Source: CAD feature listing. Evaluate the final solid. Frame: model axes, mm. A direction names the side the tool comes from. Round coordinates to 2 decimals unless told otherwise and drop trailing zeros. Order: outer loops, then holes, each group sorted by start corner. A loop starts at its lowest first (then second) coordinate and runs counter-clockwise, first axis right, second up. Notation, with made-up numbers: (30.25, 56) - (34.25, 56) arc R20 cw to (34.25, 60) - close; hole circle Ø10 at (75.5, 85.25). An arc over 180 degrees is marked (long way). Put each result on its own line as item: value. Start each with the question number.
1) Section A-A on z = 1.5. Output: boundary loops of the cut face in (x, y).
2) Access query for faces 4 (the face through (10, 25, 1)), 5 (the face through (119, 15, 5)), 6 (the face through (51, 41, 3)). Directions: +Z, -Z, +X, -X, +Y, -Y. A direction counts if a zero-diameter tool reaches every point of the face in a straight line with its end or side. Return the directions, or none.
3) Line query: probe 1 along Y at (x, z) = (174, 8.65); probe 2 along Y at (x, z) = (50, 7.75); probe 3 along X at (y, z) = (41, 4.75). Output: solid intervals per line, ascending. Write a range as [from, to].
4) Section C-C on x = 120. Output: boundary loops of the cut face in (y, z), then the cut area to 3 significant figures.
5) Section B-B on y = 26.5. Output: boundary loops of the cut face in (x, z).
6) Mould query, pull axis X, two halves, no side actions, for faces 1 (the face through (60, 41, 5)), 2 (the face through (50, 11, 1)), 3 (the face through (116, 20.5, 2)). Classes: +X half, -X half, draft (parallel to the pull), parting line (faces both ways), or undercut.
7) Section D-D on y = 42.5. Output: boundary loops of the cut face in (x, z).
8) Contact query for flat-ended pins moving along their axis: P1, Ø1.5, axis at x = 8, y = 41.5, coming from the +Z side; P2, Ø2.5, axis at x = 109, z = 2, coming from the +Y side; P3, Ø0.9, axis at x = 140, z = 1, coming from the -Y side; P4, Ø9.5, axis at x = 10, y = 9, coming from the +Z side. Output: stop coordinate, or through.
```python
from build123d import *

# Parameters (mm, degrees)
BOSS_EXTRUDE1_DEPTH = 10
SKETCH2_R           = 3
CUT_EXTRUDE1_DEPTH  = 7
SKETCH4_W           = 40
SKETCH4_H           = 40
CUT_EXTRUDE3_DEPTH  = 3
SKETCH5_R           = 1
SKETCH5_R_2         = 4
CUT_EXTRUDE4_DEPTH  = 11
SKETCH6_W           = 3
SKETCH6_H           = 3
CUT_EXTRUDE5_DEPTH  = 130
FILLET1_R           = 2
SKETCH7_R           = 1.2
CUT_EXTRUDE6_DEPTH  = 36


with BuildPart() as part:
    # Sketch1 → Boss-Extrude1 (new body)
    with BuildSketch(Plane.XY):
        Polygon((0, 0), (60, 0), (60, 15), (180, 15), (180, 35), (60, 35), (60, 50), (0, 50), align=None)
    extrude(amount=BOSS_EXTRUDE1_DEPTH)

    # Sketch2 → Cut-Extrude1 (cut)
    with BuildSketch(Plane.XY.offset(10)):
        with Locations((10, 9)):
            Circle(SKETCH2_R)
        with Locations((50, 9)):
            Circle(SKETCH2_R)
        with Locations((50, 41)):
            Circle(SKETCH2_R)
        with Locations((10, 41)):
            Circle(SKETCH2_R)
    extrude(amount=-CUT_EXTRUDE1_DEPTH, mode=Mode.SUBTRACT)

    # Sketch4 → Cut-Extrude3 (cut)
    with BuildSketch(Plane(origin=(0, 0, 0), x_dir=(-1, 0, 0), z_dir=(0, 0, -1))):
        with Locations((-30, 25)):
            Rectangle(SKETCH4_W, SKETCH4_H)
    extrude(amount=-CUT_EXTRUDE3_DEPTH, mode=Mode.SUBTRACT)

    # Sketch5 → Cut-Extrude4 (cut, through all)
    with BuildSketch(Plane(origin=(0, 0, 0), x_dir=(-1, 0, 0), z_dir=(0, 0, -1))):
        with Locations((-174, 31)):
            Circle(SKETCH5_R)
        with Locations((-174, 19)):
            Circle(SKETCH5_R)
        with Locations((-120, 25)):
            Circle(SKETCH5_R_2)
    extrude(amount=-CUT_EXTRUDE4_DEPTH, mode=Mode.SUBTRACT)

    # Sketch6 → Cut-Extrude5 (cut)
    with BuildSketch(Plane(origin=(180, 0, 0), x_dir=(0, 0, -1), z_dir=(1, 0, 0))):
        with Locations((-1.5, 31)):
            Rectangle(SKETCH6_W, SKETCH6_H)
        with Locations((-1.5, 19)):
            Rectangle(SKETCH6_W, SKETCH6_H)
    extrude(amount=-CUT_EXTRUDE5_DEPTH, mode=Mode.SUBTRACT)

    # Fillet1
    fillet1_edges = [part.edges().sort_by_distance(p)[0] for p in [
        (0, 50, 5),
        (60, 50, 5),
        (60, 0, 5),
        (0, 0, 5),
    ]]
    fillet(fillet1_edges, radius=FILLET1_R)

    # Sketch7 → Cut-Extrude6 (cut, through all)
    with BuildSketch(Plane(origin=(0, 35, 0), x_dir=(1, 0, 0), z_dir=(0, 1, 0))):
        with Locations((174, -6)):
            Circle(SKETCH7_R)
    extrude(amount=-CUT_EXTRUDE6_DEPTH, mode=Mode.SUBTRACT)


solid = part.part
```
Answer sheet:
1. outline: (0, 2) arc R2 ccw to (2, 0) - (58, 0) arc R2 ccw to (60, 2) - (60, 15) - (180, 15) - (180, 17.5) - (50, 17.5) - (50, 5) - (10, 5) - (10, 45) - (50, 45) - (50, 32.5) - (180, 32.5) - (180, 35) - (60, 35) - (60, 48) arc R2 ccw to (58, 50) - (2, 50) arc R2 ccw to (0, 48) - close; (50, 20.5) - (180, 20.5) - (180, 29.5) - (50, 29.5) - close; hole circle Ø8 at (120, 25)
2. face 4: -Z
2. face 5: +Z, -Z, +X, -Y
2. face 6: +Z
3. probe 1: [15, 18], [20, 30], [32, 35]
3. probe 2: [0, 6], [12, 38], [44, 50]
3. probe 3: [0, 7], [13, 47], [53, 60]
4. outline: (15, 0) - (17.5, 0) - (17.5, 3) - (20.5, 3) - (20.5, 0) - (21, 0) - (21, 10) - (15, 10) - close; (29, 0) - (29.5, 0) - (29.5, 3) - (32.5, 3) - (32.5, 0) - (35, 0) - (35, 10) - (29, 10) - close
4. area: 102 mm^2
5. outline: (0, 0) - (10, 0) - (10, 3) - (50, 3) - (50, 0) - (116.29, 0) - (116.29, 10) - (0, 10) - close; (123.71, 0) - (180, 0) - (180, 10) - (123.71, 10) - close; hole circle Ø2.4 at (174, 6)
6. face 1: +X half
6. face 2: undercut
6. face 3: draft
7. outline: (0, 0) - (10, 0) - (10, 3) - (7.4, 3) - (7.4, 10) - (0, 10) - close; (12.6, 3) - (47.4, 3) - (47.4, 10) - (12.6, 10) - close; (50, 0) - (60, 0) - (60, 10) - (52.6, 10) - (52.6, 3) - (50, 3) - close
8. P1: z = 3
8. P2: y = 35
8. P3: y = 15
8. P4: z = 10
